Autodesk Inventor part; units mm, degrees
ref_plane "YZ Plane" through (0, 0, 0) normal (1, 0, 0) x (0, 1, 0)
ref_plane "XZ Plane" through (0, 0, 0) normal (0, 1, 0) x (-1, 0, 0)
ref_plane "XY Plane" through (0, 0, 0) normal (0, 0, 1) x (1, 0, 0)
sketch "Sketch1" plane through (0, 0, 0) normal (0, 0, 1) x (1, 0, 0)
  line L0 (0, 0) -> (129, 0)
  line L1 (129, 0) -> (129, 85)
  line L2 (129, 85) -> (0, 85)
  line L3 (0, 85) -> (0, 0)
  line L4 (0, 85) -> (10, 85)
  line L5 (10, 85) -> (0, 0)
  line L6 (129, 85) -> (119, 85)
  line L7 (119, 85) -> (129, 0)
  dimension "d0" = 129
  dimension "d1" = 85
  dimension "d2" = 10
  dimension "d3" = 10
extrude "Extrusion1" add sketch "Sketch1" against normal blind 58 contours L5 L2 L7 L0
fillet "Fillet1" radius 4 4 edges at (5, 42.5, 0) (124, 42.5, 0) (124, 42.5, -58) (5, 42.5, -58)
shell "Shell1" thickness 3 removed faces 1 at (44.3425, 0, -19.3333)
sketch "Sketch2" plane through (0, 0, -58) normal (0, 0, -1) x (-1, 0, 0)
  line L0 (-14.0276, 85) -> (-114.9724, 85)
  line L1 (-124.9724, 0) -> (-4.0276, 0)
  line L2 (-22.0276, 0) -> (-22.0276, 55)
  line L3 (-22.0276, 55) -> (-22.0276, 55)
  circle A0 centre (-22.0276, 55) radius 7.829
  line L4 (-29.8566, 55) -> (-36.5566, 55)
  line L5 (-36.5566, 55) -> (-44.4066, 55)
  circle A1 centre (-44.4066, 55) radius 7.85
  line L6 (-52.2566, 55) -> (-87.7566, 55)
  circle A2 centre (-87.7566, 55) radius 22.5
  line L7 (-4.0276, 0) -> (-22.0276, 0)
  point P0 (0, 0)
  dimension "d10" = 15.6579
  dimension "d8" = 55
  dimension "d9" = 0
  dimension "d11" = 6.7
  dimension "d12" = 7.85
  dimension "d13" = 35.5
  dimension "d14" = 45
  dimension "d15" = 18
extrude "Extrusion2" cut sketch "Sketch2" against normal blind 5
chamfer "Chamfer1" distance 3 distance2 1 1 edges at (110.2566, 55, -58) measured on face at (69.5927, 11.3207, -58)
properties part number "Box MKIV Version 1"
Source: CAD feature listing. Evaluate the final solid. Frame: model axes, mm. A direction names the side the tool comes from. Give positions to 0.01 mm unless a question says otherwise; leave off trailing zeros. Loops run counter-clockwise (first coordinate to the right, second up) from the corner with the lowest first, then second, coordinate; pieces in that order, holes last. Notation, with made-up numbers: (-2, 60) -> (9, 60) arc R17 ccw to (9, 80) -> close; hole circle Ø6 at (48.5, 54.5). An arc over 180 degrees is marked (long way). Use a Markdown table: item, result. Add a question column.
1) Line query: line 1 along Z through (x, y) = (108.5, 14.5); line 2 along Y through (x, z) = (84.5, -40); line 3 along X through (y, z) = (64.5, -13). Output: solid intervals per line, ascending. Write a range as [from, to].
2) First-contact query: pin 1 (12 mm diameter, centred on y = 16, z = -14, fed in from -X); pin 2 (3 mm diameter, centred on x = 43, z = -16.5, fed in from -Y); pin 3 (3 mm diameter, centred on y = 55.5, z = -33.5, fed in from -X). Flat tips, straight axial feed; report the tip coordinate or a pass-through.
3) Reachability of faces 1 (the face through (64, 32, -55)), 2 (the face through (122.85, 41.99, -56.86)), 3 (the face through (29.85, 55.34, -56.52)) from +Z, -Z, +X, -X, +Y, -Y: full face, straight path, thin tool, end or side. Return the list, or none.
4) Section query B-B, the plane x = 40. Return the cut outline in (y, z), then the cut area to 3 significant figures.
5) Section query C-C, the plane y = 55. Count the separate pieces of the cut face and the enclosed holes in it, then the cut area to 3 significant figures.
6) Pull-direction query (Z, two-part tool) for faces 4 (the face through (64, 34, -58)), 5 (the face through (59, 0, -57)), 6 (the face through (7.91, 41.57, -28.65)); classes: +Z half, -Z half, draft (parallel to the pull), parting line (faces both ways), or undercut.
7) Section query A-A, the plane z = -36. Return the cut outline in (x, y).
Numbers:
| question | item | result |
|---|---|---|
| 1 | line 1 | z = [-58, -55], [-3, 0] |
| 1 | line 2 | y = [82, 85] |
| 1 | line 3 | x = [7.59, 10.61], [118.39, 121.41] |
| 2 | pin 1 | stops at x = 1.18 |
| 2 | pin 2 | stops at y = 82 |
| 2 | pin 3 | stops at x = 6.35 |
| 3 | face 1 | -Y |
| 3 | face 2 | -Z, +X, +Y |
| 3 | face 3 | -Z |
| 4 | outline | (0, -58) -> (48.5, -58) -> (48.5, -55) -> (0, -55) -> close; (0, -3) -> (82, -3) -> (82, -55) -> (61.5, -55) -> (61.5, -58) -> (85, -58) -> (85, 0) -> (0, 0) -> close |
| 4 | area | 627 mm2 |
| 5 | separate pieces | 3 |
| 5 | enclosed holes | 0 |
| 5 | area | 765 mm2 |
| 6 | face 4 | -Z half |
| 6 | face 5 | draft |
| 6 | face 6 | undercut |
| 7 | outline | (0, 0) -> (3.02, 0) -> (12.67, 82) -> (116.33, 82) -> (125.98, 0) -> (129, 0) -> (119, 85) -> (10, 85) -> close |
